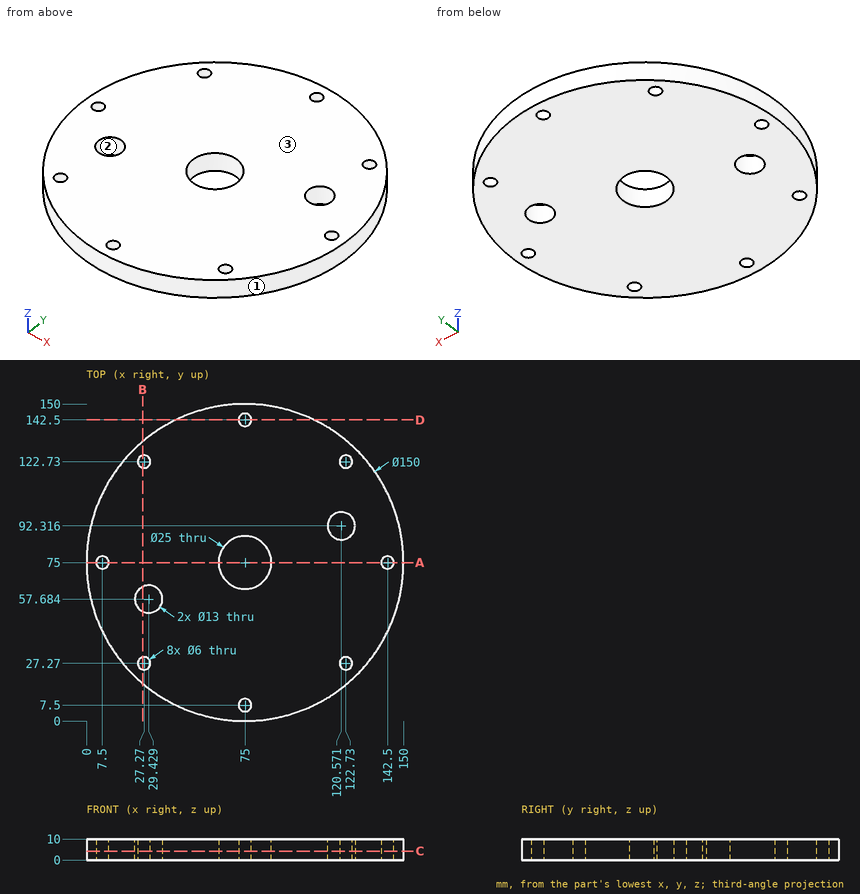
Verification items for this drawing (mm, ordinates from the low corner). Coordinates: 2 decimals unless noted, no trailing zeros. Write each loop counter-clockwise with the first axis right and the second up, starting at its lowest first coordinate (ties: lowest second). Pieces come first, ordered by that corner, then holes. Notation, with made-up numbers: (-22, 9) -> (11, 9) arc R23 ccw to (11, 41) -> close; hole circle Ø8 at (15, 39). An arc over 180 degrees is marked (long way). One line per item, written item: value. Start each with the question number.
Q1. Cross-section at B-B on x = 26.5. Enter the section's corners in (y, z).
Q2. Mould release check, pull along X, two halves, no side actions. Record for the marked faces 1, 2 and 3: pulls with the +X half, pulls with the -X half, needs draft (parallel to the pull), parting line crosses it, or undercut.
Q3. Cross-section at D-D on y = 142.5. Enter the section's corners in (x, z), and give its area (3 significant figures).
Q4. Cross-section at A-A on y = 75. Enter the section's corners in (x, z), and give its area (3 significant figures).
Q5. Cross-section at C-C on z = 4.25. State how many separate pieces and enclosed holes the cut face has, and give its area (3 significant figures).
Q6. Go/stop test with flat-tipped pins: P1, Ø5, axis at x = 27.27, y = 122.73, coming from the -Z side; P2, Ø3, axis at y = 20, z = 3.5, coming from the -X side; P3, Ø6, axis at y = 99, z = 4.5, coming from the +X side; P4, Ø1.5, axis at x = 59, z = 8.5, coming from the -Y side. Record where each tip stops, or that it passes through.
Q7. Thickness scan on L1, parallel to Y at x = 75, z = 3.5; L2, parallel to Y at x = 34, z = 3.5 (1 decimal); L3, parallel to Y at x = 66.5, z = 5.75 (1 decimal). Record the ranges inside material, lowest first. Write a range as from..to.
Checked values:
1. outline: (17.79, 0) -> (24.37, 0) -> (24.37, 10) -> (17.79, 10) -> close; (30.17, 0) -> (51.88, 0) -> (51.88, 10) -> (30.17, 10) -> close; (63.49, 0) -> (119.83, 0) -> (119.83, 10) -> (63.49, 10) -> close; (125.63, 0) -> (132.21, 0) -> (132.21, 10) -> (125.63, 10) -> close
2. face 1: parting line crosses it
2. face 2: undercut
2. face 3: needs draft
3. outline: (42.31, 0) -> (72, 0) -> (72, 10) -> (42.31, 10) -> close; (78, 0) -> (107.69, 0) -> (107.69, 10) -> (78, 10) -> close
3. area: 594 mm²
4. outline: (0, 0) -> (4.5, 0) -> (4.5, 10) -> (0, 10) -> close; (10.5, 0) -> (62.5, 0) -> (62.5, 10) -> (10.5, 10) -> close; (87.5, 0) -> (139.5, 0) -> (139.5, 10) -> (87.5, 10) -> close; (145.5, 0) -> (150, 0) -> (150, 10) -> (145.5, 10) -> close
4. area: 1,130 mm²
5. separate pieces: 1
5. enclosed holes: 11
5. area: 16,700 mm²
6. P1: passes through
6. P2: stops at x = 22.44
6. P3: stops at x = 147
6. P4: stops at y = 1.57
7. L1: y = 0..4.5, 10.5..62.5, 87.5..139.5, 145.5..150
7. L2: y = 12.2..53.1, 62.3..137.8
7. L3: y = 0.5..65.8, 84.2..149.5
